Design review of the part built by this model. Coordinates are the model's own, in mm. A direction names the side the tool comes from. Coordinates: 2 decimals unless noted, no trailing zeros. Write each loop counter-clockwise with the first axis right and the second up, starting at its lowest first coordinate (ties: lowest second). Pieces come first, ordered by that corner, then holes.
Q1. Take a section at A-A, the plane z = 12.25. Write out the cut boundary in (x, y) (3 decimals).
Q2. For pin 1 Ø10 at (x, z) = (-5.5, 15.5) entering from -Y; pin 2 Ø4 at (x, z) = (4.5, 3) entering from +Y; pin 3 Ø1.5 at (y, z) = (-7, 7.5) entering from +X, all flat-tipped, find the tip position at first contact; note any pin that passes through.
Q3. For faces 4 (the cylindrical face through (-8.2, -7.52, 16.23)), 5 (the flat face through (0, 4, 0)), 6 (the flat face through (1, -1, 0.25)), list the 3-axis set-ups (+Z, -Z, +X, -X, +Y, -Y) from which the entire face can be reached by the end or side of a thin tool; tool diameter is ignored.
Q4. For L1, parallel to Z at x = -6.5, y = -13.5; L2, parallel to Z at x = -2, y = -3; L3, parallel to X at y = 6, z = 3, list the stretches that pass through material, from the lowest coordinate up.
Q5. The part is to be moulded in two halves that separate along Y. For faces 1 (the flat face through (-10, -6, 15)), 2 (the cylindrical face through (-2.79, 12.57, 9.93)), 3 (the flat face through (-5.15, -5.53, 0.13)), say which applies: released by +Y, released by -Y, zero draft, split by the parting line, or undercut.
Autodesk Inventor part; units mm, degrees
ref_plane "YZ Plane" through (0, 0, 0) normal (1, 0, 0) x (0, 1, 0)
ref_plane "XZ Plane" through (0, 0, 0) normal (0, 1, 0) x (-1, 0, 0)
ref_plane "XY Plane" through (0, 0, 0) normal (0, 0, 1) x (1, 0, 0)
sketch "Sketch1" plane through (0, 0, 0) normal (0, 0, 1) x (1, 0, 0)
  circle A0 centre (0, 0) radius 11.125
  circle A1 centre (0, 0) radius 12.875
  circle A2 centre (0, 0) radius 17.875
  dimension "d0" = 22.25
  dimension "d1" = 25.75
  dimension "d2" = 5
extrude "Extrusion1" add sketch "Sketch1" along normal blind 5 contours A0 | A1 | A2
extrude "Extrusion2" add sketch "Sketch1" along normal blind 10 from surface at 5 contours A0 | A1
extrude "Extrusion3" add sketch "Sketch1" along normal blind 2.5 from surface at 15 contours A0
fillet "Fillet1" radius 1.25 1 edges at (-17.875, 0, 0)
sketch "Sketch2" plane through (0, 0, 0) normal (0, 0, -1) x (-1, 0, 0)
  line L0 (-12.5, -12.5) -> (12.5, -12.5)
  line L1 (12.5, -12.5) -> (12.5, 12.5)
  line L2 (12.5, 12.5) -> (-12.5, 12.5)
  line L3 (-12.5, 12.5) -> (-12.5, -12.5)
  line L4 (-12.5, -12.5) -> (12.5, 12.5) construction
  line L5 (12.5, -12.5) -> (-12.5, 12.5) construction
  line L6 (-12.5, 12.5) -> (12.5, 12.5) construction
  line L7 (12.5, 12.5) -> (12.5, -12.5) construction
  line L8 (12.5, -12.5) -> (-12.5, -12.5) construction
  line L9 (-12.5, -12.5) -> (-12.5, 12.5) construction
  line L10 (8.9708, -10) -> (5.5186, -10)
  line L11 (5.5186, -10) -> (-0.8023, -2.0421)
  line L12 (-0.8023, -2.0421) -> (-3.8493, -2.0421)
  line L13 (-3.8493, -2.0421) -> (-3.8493, -10)
  line L14 (-3.8493, -10) -> (-6.5073, -10)
  line L15 (-6.5073, -10) -> (-6.5073, 10)
  line L16 (-6.5073, 10) -> (-1.3533, 10)
  spline S0 degree 2 poles (-1.3533, 10) (0.3647, 10) (2.6823, 9.6272) (3.7358, 8.9465) knots 0 0 0 1 2 2 2
  spline S1 degree 2 poles (3.7358, 8.9465) (4.7893, 8.2658) (6.0049, 6.1426) (6.0049, 4.5705) knots 0 0 0 1 2 2 2
  spline S2 degree 2 poles (6.0049, 4.5705) (6.0049, 2.3825) (3.7682, -0.5835) (1.8558, -1.2966) knots 0 0 0 1 2 2 2
  line L17 (1.8558, -1.2966) -> (8.9708, -10)
  spline S3 degree 2 poles (3.2334, 4.3598) (3.2334, 5.235) (2.6175, 6.5802) (1.9692, 7.0178) knots 0 0 0 1 2 2 2
  spline S4 degree 2 poles (1.9692, 7.0178) (1.4019, 7.3906) (-0.1053, 7.6985) (-1.2075, 7.6985) knots 0 0 0 1 2 2 2
  line L18 (-1.2075, 7.6985) -> (-3.8493, 7.6985)
  line L19 (-3.8493, 7.6985) -> (-3.8493, 0.1783)
  line L20 (-3.8493, 0.1783) -> (-1.5154, 0.1783)
  spline S5 degree 2 poles (-1.5154, 0.1783) (-0.3647, 0.1783) (1.4668, 0.5835) (2.0989, 1.2156) knots 0 0 0 1 2 2 2
  spline S6 degree 2 poles (2.0989, 1.2156) (2.6823, 1.7666) (3.2334, 3.3225) (3.2334, 4.3598) knots 0 0 0 1 2 2 2
  point P0 (0, 0)
  dimension "d10" = 25
  dimension "d11" = 25
extrude "Extrusion4" cut sketch "Sketch2" against normal blind 0.25 contours L10 L11 L12 L13 L14 L15 L16 S0 S1 S2 L17
chamfer "Chamfer1" distance 0.25 angle 45 18 edges at (-7.2447, -10, 0.25) (-2.3582, -6.0211, 0.25) (2.3258, -2.0421, 0.25) (3.8493, -6.0211, 0.25) (5.1783, -10, 0.25) (6.5073, 0, 0.25) (3.9303, 10, 0.25) (-1.5235, 9.8136, 0.25) (-5.3971, 7.2042, 0.25) (-4.8865, 0.8995, 0.25) (-5.4133, -5.6483, 0.25) (-2.9579, 2.5446, 0.25) (-2.9254, 5.9076, 0.25) (-0.6483, 7.5446, 0.25) (2.5284, 7.6985, 0.25) (3.8493, 3.9384, 0.25) (2.6823, 0.1783, 0.25) (-0.5511, 0.3809, 0.25)
properties part number "SM1 Removal Tool"
Responses:
1. outline: circle Ø25.75 at (0, 0)
2. pin 1: stops at y = -12.86
2. pin 2: stops at y = 17.7
2. pin 3: stops at x = 11.26
3. face 4: +Z
3. face 5: -Z, +X, -X, +Y, -Y
3. face 6: -Z
4. L1: z = 0 to 5
4. L2: z = 0.25 to 17.5
4. L3: x = -16.84 to 16.84
5. face 1: zero draft
5. face 2: split by the parting line
5. face 3: undercut
